from build123d import *

# Parameters (mm, degrees)
SKETCH1_R           = 4.75
BOSS_EXTRUDE1_DEPTH = 10
SKETCH2_R           = 10
BOSS_EXTRUDE2_DEPTH = 5
SKETCH3_R           = 4.75
BOSS_EXTRUDE3_DEPTH = 13.2
SKETCH4_R           = 4.75
CUT_EXTRUDE1_DEPTH  = 5


with BuildPart() as part:
    # Sketch1 → Boss-Extrude1 (new body)
    with BuildSketch(Plane(origin=(0, 0, 0), x_dir=(1, 0, 0), z_dir=(0, 1, 0))):
        Circle(SKETCH1_R)
    extrude(amount=BOSS_EXTRUDE1_DEPTH)

    # Sketch2 → Boss-Extrude2 (add)
    with BuildSketch(Plane(origin=(0, 10, 0), x_dir=(1, 0, 0), z_dir=(0, 1, 0))):
        Circle(SKETCH2_R)
    extrude(amount=BOSS_EXTRUDE2_DEPTH)

    # Sketch3 → Boss-Extrude3 (add)
    with BuildSketch(Plane.XZ):
        Circle(SKETCH3_R)
    extrude(amount=BOSS_EXTRUDE3_DEPTH)

    # Sketch4 → Cut-Extrude1 (cut)
    with BuildSketch(Plane.XZ.offset(13.2)):
        Circle(SKETCH4_R)
    extrude(amount=-CUT_EXTRUDE1_DEPTH, mode=Mode.SUBTRACT)


solid = part.part
Could you check a few things on this model? Use its own coordinates, in mm. A direction names the side the tool comes from. Round coordinates to 2 decimals unless told otherwise and drop trailing zeros. Order: outer loops, then holes, each group sorted by start corner. A loop starts at its lowest first (then second) coordinate and runs counter-clockwise, first axis right, second up.
Q1. Imagine slicing it at C-C, the plane y = 1.75. List the corners of the cut face in (x, z) for me.
Geometry says:
outline: circle Ø9.5 at (0, 0)
Q2. Imagine slicing it at D-D, the plane z = -6.5. List the corners of the cut face in (x, y) for me, then the cut area to 3 significant figures.
Geometry says:
outline: (-7.6, 10) - (7.6, 10) - (7.6, 15) - (-7.6, 15) - close
area: 76.0 mm2
Q3. Which directions (+Z, -Z, +X, -X, +Y, -Y) give clear straight access to the entire face, cutting with the end or side of a thin tool? Please do faces 1 (the face through (-2.17, 12.46, 9.76)), 2 (the face through (-2.4, 10, 4.3)).
Geometry says:
face 1: +Y, -Y
face 2: -Y
Q4. Imagine slicing it at B-B, the plane x = 0. List the corners of the cut face in (y, z) for me, then the cut area to 3 significant figures.
Geometry says:
outline: (-8.2, -4.75) - (10, -4.75) - (10, -10) - (15, -10) - (15, 10) - (10, 10) - (10, 4.75) - (-8.2, 4.75) - close
area: 273 mm2
Q5. Imagine slicing it at A-A, the plane z = 0. List the corners of the cut face in (x, y) for me, then the cut area to 3 significant figures.
Geometry says:
outline: (-10, 10) - (-4.75, 10) - (-4.75, -8.2) - (4.75, -8.2) - (4.75, 10) - (10, 10) - (10, 15) - (-10, 15) - close
area: 273 mm2
Q6. I'm going to push flat-ended pins straight in: P1, Ø4, axis at y = 5.5, z = 7, coming from the +X side; P2, Ø2, axis at y = 4, z = -1, coming from the -X side. Where does each tip first touch, or does it pass through?
Geometry says:
P1: passes through
P2: stops at x = -4.75
Q7. Please list where these lines run through material, in increasing order: probe 1 along Y at (x, z) = (6, -7.5); probe 2 along X at (y, z) = (4.5, -3.75); probe 3 along Z at (x, y) = (2.5, 2.5).
Geometry says:
probe 1: y = 10 to 15
probe 2: x = -2.92 to 2.92
probe 3: z = -4.04 to 4.04
